```python
from build123d import *

# Parameters (mm, degrees)
EXTRU_MINCE1_DEPTH = 26
EXTRUSION1_REACH   = 29
ESQUISSE4_R        = 3
ESQUISSE5_R        = 1.5
EXTRUSION2_DEPTH   = 2


with BuildPart() as part:
    # Esquisse1 → Extru.-Mince1 (new body)
    with BuildSketch(Plane.XY):
        Polygon((-8, 0), (0, 0), (0, 25), (23, 25), (23, 0), (31, 0), (31, 2), (25, 2), (25, 27), (-2, 27), (-2, 2), (-8, 2), align=None)
    extrude(amount=EXTRU_MINCE1_DEPTH)

    # Esquisse4 → Extrusion1 (cut, up to next)
    with BuildSketch(Plane(origin=(0, 27, 0), x_dir=(1, 0, 0), z_dir=(0, 1, 0)), mode=Mode.PRIVATE) as extrusion1_sk1:
        with Locations((11.5, -13)):
            Circle(ESQUISSE4_R)
    extrusion1_tool1 = extrude(extrusion1_sk1.sketch, amount=-EXTRUSION1_REACH, mode=Mode.PRIVATE) & part.part
    add(extrusion1_tool1.solids().sort_by_distance((11.5, 27, 13))[0], mode=Mode.SUBTRACT)

    # Esquisse5 → Extrusion2 (cut)
    with BuildSketch(Plane(origin=(0, 2, 0), x_dir=(1, 0, 0), z_dir=(0, 1, 0))):
        with Locations((-5, -21)):
            Circle(ESQUISSE5_R)
        with Locations((-5, -5)):
            Circle(ESQUISSE5_R)
    extrusion2 = extrude(amount=-EXTRUSION2_DEPTH, mode=Mode.SUBTRACT)

    # Sym_trie1: Extrusion2 across plane
    add(extrusion2.mirror(Plane(origin=(11.5, 27, 26), x_dir=(0, 0, 1), z_dir=(-1, 0, 0))), mode=Mode.SUBTRACT)


solid = part.part
```
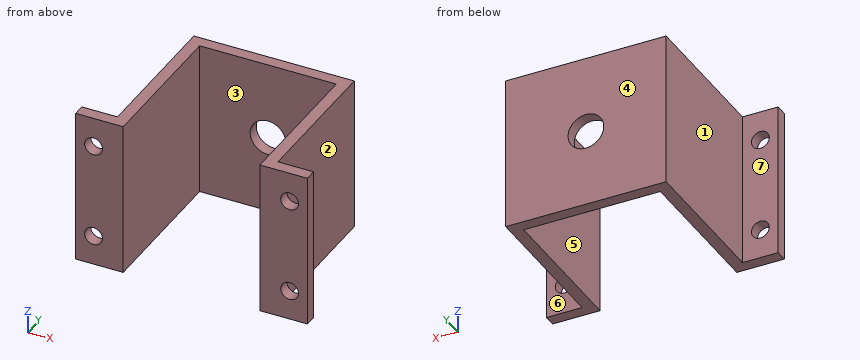
Model file for the job. Use its own axes, mm. Face numbers are marked on the shaded views. A direction names the side the tool comes from. Coordinates: 2 decimals unless noted, no trailing zeros. Order: outer loops, then holes, each group sorted by start corner. A loop starts at its lowest first (then second) coordinate and runs counter-clockwise, first axis right, second up. Notation, with made-up numbers: (-20, -30) - (14, -30) arc R11 cw to (14, -24) - close; hole circle Ø9 at (-19.75, 30.5). An arc over 180 degrees is marked (long way). Return JSON: item names as keys, results as strings. Group by question number.
1) Flat gauge pins, fed straight in: P1, Ø12.5, axis at y = 14.5, z = 7.5, coming from the -X side; P2, Ø7, axis at x = 17, z = 14.5, coming from the -Y side; P3, Ø5, axis at y = 15.5, z = 20.5, coming from the +X side. Where does each tip first touch, or does it go through?
2) Saw through at A-A, the plane z = 5. Write the cut outline in (x, y), plus the area to 3 significant figures.
3) Tool access for the marked faces 5, 6 and 7: list every direction of +Z, -Z, +X, -X, +Y, -Y with a clear straight run to the whole face (end or side of a thin tool).
4) Probe line 1 (Z direction, x = 28, y = 0.8); line 2 (X direction, y = 1.3, z = 21); line 3 (X direction, y = 13, z = 19). List the from-to ranges inside material, lowest first. Write a range as from..to.
5) Saw through at D-D, the plane y = 14. Write the cut outline in (x, z).
6) Saw through at B-B, the plane x = 11.5. Write the cut outline in (y, z), plus the area to 3 significant figures.
7) Mould opens along X. For the marked faces 1, 2, 3 and 4 say: released by +X, released by -X, zero draft, split by the parting line, or undercut.
8) Saw through at C-C, the plane z = 13. Write the cut outline in (x, y), plus the area to 3 significant figures.
Values found:
{
 "1": {"P1": "stops at x = -2", "P2": "stops at y = 25", "P3": "stops at x = 25"},
 "2": {"outline": "(-8, 0) - (-6.5, 0) - (-6.5, 2) - (-8, 2) - close; (-3.5, 0) - (0, 0) - (0, 25) - (23, 25) - (23, 0) - (26.5, 0) - (26.5, 2) - (25, 2) - (25, 27) - (-2, 27) - (-2, 2) - (-3.5, 2) - close; (29.5, 0) - (31, 0) - (31, 2) - (29.5, 2) - close", "area": "166 mm²"},
 "3": {"face 5": "+Z, -Z, -Y", "face 6": "+Z, -Z, +X, +Y", "face 7": "+Z, -Z, -X, +Y"},
 "4": {"line 1": "z = 0..3.5, 6.5..19.5, 22.5..26", "line 2": "x = -8..-6.5, -3.5..0, 23..26.5, 29.5..31", "line 3": "x = -2..0, 23..25"},
 "5": {"outline": "(-2, 0) - (0, 0) - (0, 26) - (-2, 26) - close; (23, 0) - (25, 0) - (25, 26) - (23, 26) - close"},
 "6": {"outline": "(25, 0) - (27, 0) - (27, 10) - (25, 10) - close; (25, 16) - (27, 16) - (27, 26) - (25, 26) - close", "area": "40.0 mm²"},
 "7": {"face 1": "released by -X", "face 2": "released by +X", "face 3": "undercut", "face 4": "zero draft"},
 "8": {"outline": "(-8, 0) - (0, 0) - (0, 25) - (8.5, 25) - (8.5, 27) - (-2, 27) - (-2, 2) - (-8, 2) - close; (14.5, 25) - (23, 25) - (23, 0) - (31, 0) - (31, 2) - (25, 2) - (25, 27) - (14.5, 27) - close", "area": "166 mm²"}
}
